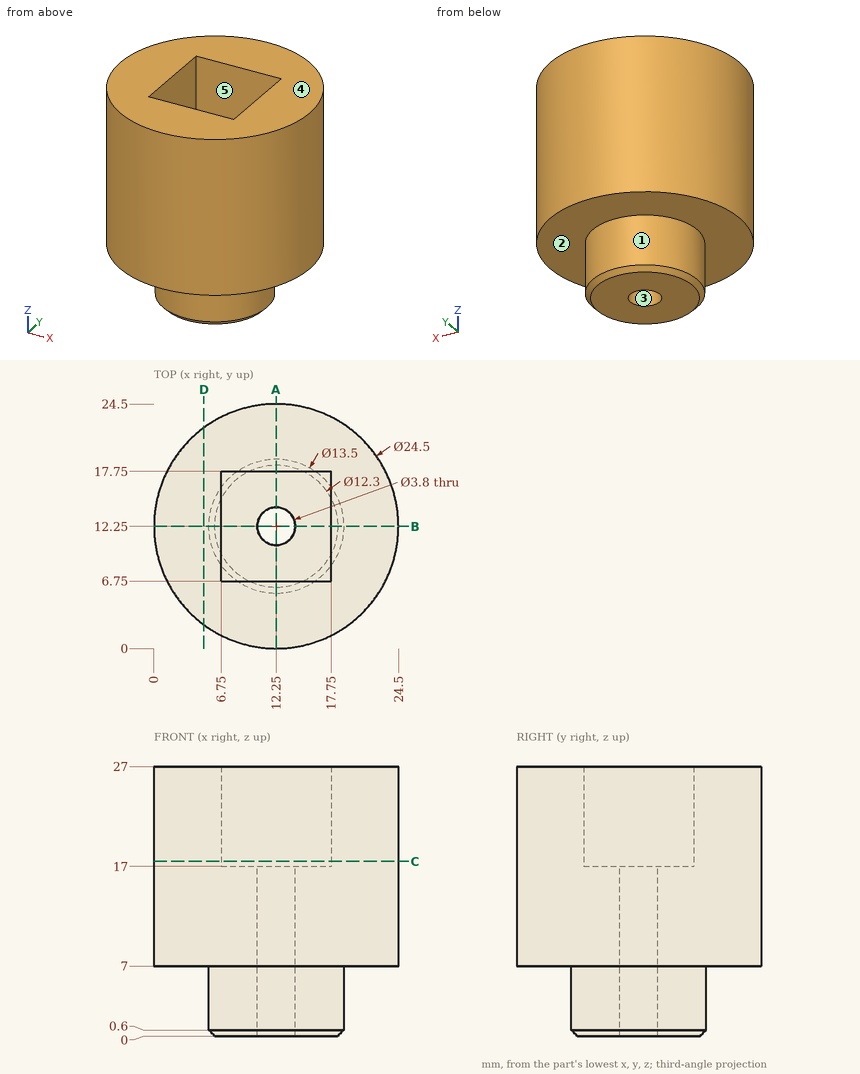
Part print with two shaded views. Sizes in mm from the minimum x, y, z corner. A direction names the side the tool comes from. Coordinates: 2 decimals unless noted, no trailing zeros. Loops run counter-clockwise (first coordinate to the right, second up) from the corner with the lowest first, then second, coordinate; pieces in that order, holes last. Notation, with made-up numbers: (38, -13.5) -> (80, -13.5) arc R24 ccw to (80, 20.5) -> close; hole circle Ø9 at (-36.75, 53). An arc over 180 degrees is marked (long way). Answer as a JSON object with one key per item and string values.
Q1. Cut at A-A (x = 12.25). List the corners of the cut face in (y, z), and give its area (3 significant figures).
Report:
{"outline": "(0, 7) -> (5.5, 7) -> (5.5, 0.6) -> (6.1, 0) -> (10.35, 0) -> (10.35, 17) -> (6.75, 17) -> (6.75, 27) -> (0, 27) -> close; (14.15, 0) -> (18.4, 0) -> (19, 0.6) -> (19, 7) -> (24.5, 7) -> (24.5, 27) -> (17.75, 27) -> (17.75, 17) -> (14.15, 17) -> close", "area": "410 mm2"}
Q2. 3-axis set-ups, long thin cutter, end or side, ignore diameter. For the marked faces 4 and 5: which of +Z, -Z, +X, -X, +Y, -Y reach the whole face in a straight line?
Report:
{"face 4": "+Z, +X, -X, +Y, -Y", "face 5": "+Z"}
Q3. Probe probe 1 along Y at (x, z) = (12.25, 17.25); probe 2 along Y at (x, z) = (12.25, 6.5); probe 3 along Z at (x, y) = (8, 20.75). List the from-to ranges inside material, lowest first.
Report:
{"probe 1": "y = 0 to 6.75, 17.75 to 24.5", "probe 2": "y = 5.5 to 10.35, 14.15 to 19", "probe 3": "z = 7 to 27"}
Q4. Cut at D-D (x = 5). List the corners of the cut face in (y, z), and give its area (3 significant figures).
Report:
{"outline": "(2.38, 7) -> (22.12, 7) -> (22.12, 27) -> (2.38, 27) -> close", "area": "395 mm2"}
Q5. Pull direction X, two halves, no side cores. Call the marked faces 1, 2 and 3: released by +X, released by -X, zero draft, split by the parting line, or undercut.
Report:
{"face 1": "split by the parting line", "face 2": "zero draft", "face 3": "undercut"}
Q6. Cut at C-C (z = 17.5). List the corners of the cut face in (x, y), and give its area (3 significant figures).
Report:
{"outline": "circle Ø24.5 at (12.25, 12.25); hole (6.75, 6.75) -> (17.75, 6.75) -> (17.75, 17.75) -> (6.75, 17.75) -> close", "area": "350 mm2"}
Q7. Flat gauge pins, fed straight in: P1, Ø1.5, axis at x = 10, z = 20.5, coming from the -Y side; P2, Ø12, axis at x = 6, z = 13.5, coming from the -Y side; P3, Ø5.5, axis at x = 12.5, y = 14, coming from the +Z side; P4, Ø2.5, axis at x = 12.25, y = 12.25, coming from the -Z side. Where does each tip first touch, or does it go through?
Report:
{"P1": "stops at y = 0.09", "P2": "stops at y = 0", "P3": "stops at z = 17", "P4": "passes through"}
